The figure shows three views and two pictorial views of one solid part (mm, origin at its lowest corner). Answer the questions. Coordinates: 2 decimals unless noted, no trailing zeros. Order: outer loops, then holes, each group sorted by start corner. A loop starts at its lowest first (then second) coordinate and runs counter-clockwise, first axis right, second up. Notation, with made-up numbers: (-26.5, 48) -> (1.5, 48) arc R25 cw to (1.5, 87) -> close; hole circle Ø1 at (43, -18). An arc over 180 degrees is marked (long way). Return JSON: item names as keys, results as strings.
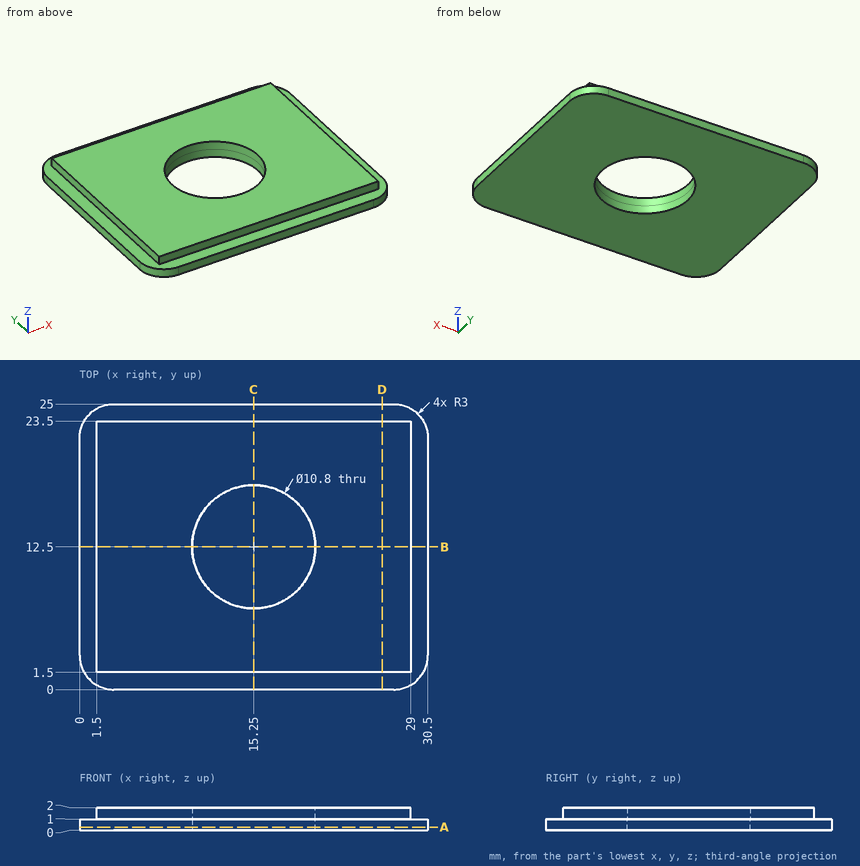
1. The part is cut by section A-A on z = 0.3. Give the vertices of the cut face in (x, y).
Answer block:
{"outline": "(0, 3) arc R3 ccw to (3, 0) -> (27.5, 0) arc R3 ccw to (30.5, 3) -> (30.5, 22) arc R3 ccw to (27.5, 25) -> (3, 25) arc R3 ccw to (0, 22) -> close; hole circle Ø10.8 at (15.25, 12.5)"}
2. The part is cut by section C-C on x = 15.25. Give the vertices of the cut face in (y, z), and give its area (3 significant figures).
Answer block:
{"outline": "(0, 0) -> (7.1, 0) -> (7.1, 2) -> (1.5, 2) -> (1.5, 1) -> (0, 1) -> close; (17.9, 0) -> (25, 0) -> (25, 1) -> (23.5, 1) -> (23.5, 2) -> (17.9, 2) -> close", "area": "25.4 mm2"}
3. The part is cut by section B-B on y = 12.5. Give the vertices of the cut face in (x, z), and give its area (3 significant figures).
Answer block:
{"outline": "(0, 0) -> (9.85, 0) -> (9.85, 2) -> (1.5, 2) -> (1.5, 1) -> (0, 1) -> close; (20.65, 0) -> (30.5, 0) -> (30.5, 1) -> (29, 1) -> (29, 2) -> (20.65, 2) -> close", "area": "36.4 mm2"}
4. The part is cut by section D-D on x = 26.5. Give the vertices of the cut face in (y, z), and give its area (3 significant figures).
Answer block:
{"outline": "(0, 0) -> (25, 0) -> (25, 1) -> (23.5, 1) -> (23.5, 2) -> (1.5, 2) -> (1.5, 1) -> (0, 1) -> close", "area": "47.0 mm2"}
5. Each of these flat-tipped pins is pushed along its axis until it touches: pin 1 Ø0.8 at (y, z) = (10, 1.5) entering from -X; pin 2 Ø0.5 at (y, z) = (16, 1.5) entering from +X. Where does it stop, or does it pass through?
Answer block:
{"pin 1": "stops at x = 1.5", "pin 2": "stops at x = 29"}
6. Consider line 1 (X direction, y = 12.5, z = 1.8); line 2 (X direction, y = 12.5, z = 0.65); line 3 (Y direction, x = 15.25, z = 1.45). Determine where each line is inside the solid, lowest interval first. Write a range as from..to.
Answer block:
{"line 1": "x = 1.5..9.85, 20.65..29", "line 2": "x = 0..9.85, 20.65..30.5", "line 3": "y = 1.5..7.1, 17.9..23.5"}
